from build123d import *

# Parameters (mm, degrees)
SKETCH3_W          = 28
SKETCH3_H          = 28
CUT_EXTRUDE1_DEPTH = 4


with BuildPart() as part:
    # Sketch1 → Revolve1 (revolve)
    with BuildSketch(Plane.XY):
        Polygon((0, 0), (0, 6.9), (0.511348244, 9.8), (3.488651756, 9.8), (4, 6.9), (4, 0), align=None)
    revolve(axis=Axis((4, 0, 0), (-1, 0, 0)))

    # Sketch2 → Cut-Revolve1 (revolve, cut)
    with BuildSketch(Plane.XY):
        Polygon((0, 0), (0, 6), (0.5415, 5.4585), (3.4585, 5.4585), (4, 6), (4, 0), align=None)
    revolve(axis=Axis((4, 0, 0), (-1, 0, 0)), mode=Mode.SUBTRACT)

    # Sketch3 → Cut-Extrude1 (cut)
    with BuildSketch(Plane(origin=(0, 0, 0), x_dir=(0, 0, -1), z_dir=(1, 0, 0))):
        Rectangle(SKETCH3_W, SKETCH3_H)
        Polygon((-7, -4.041451884), (0, -8.082903769), (7, -4.041451884), (7, 4.041451884), (0, 8.082903769), (-7, 4.041451884), align=None, mode=Mode.SUBTRACT)
    extrude(amount=CUT_EXTRUDE1_DEPTH, mode=Mode.SUBTRACT)


solid = part.part
Design review of the part built by this model. Coordinates are the model's own, in mm. Coordinates: 2 decimals unless noted, no trailing zeros. Order: outer loops, then holes, each group sorted by start corner. A loop starts at its lowest first (then second) coordinate and runs counter-clockwise, first axis right, second up.
Item 1: Take a section at A-A, the plane y = 0. Write out the cut boundary in (x, z), then the cut area to 3 significant figures.
Item 2: For line 1 (Z direction, x = 2.25, y = 0); line 2 (Y direction, x = 3.85, z = -2.5); line 3 (Y direction, x = 2.15, z = -1.5), list the stretches that pass through material, from the lowest coordinate up.
Item 3: For pin 1 Ø2 at (x, y) = (1, 6) entering from +Z; pin 2 Ø1.5 at (y, z) = (-5, -1) entering from +X, all flat-tipped, find the tip position at first contact; note any pin that passes through.
Item 4: Take a section at B-B, the plane x = 0.95. Write out the cut boundary in (y, z), then the cut area to 3 significant figures.
The answers:
1. outline: (0, -6.9) - (0.02, -7) - (3.98, -7) - (4, -6.9) - (4, -6) - (3.46, -5.46) - (0.54, -5.46) - (0, -6) - close; (0, 6) - (0.54, 5.46) - (3.46, 5.46) - (4, 6) - (4, 6.9) - (3.98, 7) - (0.02, 7) - (0, 6.9) - close
1. area: 11.7 mm2
2. line 1: z = -7 to -5.46, 5.46 to 7
2. line 2: y = -6.64 to -5.29, 5.29 to 6.64
2. line 3: y = -7.22 to -5.25, 5.25 to 7.22
3. pin 1: stops at z = 5.34
3. pin 2: stops at x = 3.85
4. outline: (-8.08, 0) - (-4.04, -7) - (4.04, -7) - (8.08, 0) - (4.04, 7) - (-4.04, 7) - close; hole circle Ø10.92 at (0, 0)
4. area: 76.1 mm2
